from build123d import *

# Parameters (mm, degrees)
SKETCH1_R           = 9.8
SKETCH1_R_2         = 5
BOSS_EXTRUDE1_DEPTH = 10
SKETCH2_W           = 11.3
SKETCH2_H           = 11.3
CUT_EXTRUDE1_DEPTH  = 5
SKETCH3_W           = 11.313408722
SKETCH3_H           = 4.707055676
CUT_EXTRUDE2_DEPTH  = 3
SKETCH4_W           = 5.404805584
SKETCH4_H           = 18.076359344
SKETCH4_W_2         = 5.663408722
SKETCH4_H_2         = 17.947057775
CUT_EXTRUDE3_DEPTH  = 3
CHAMFER1_SIZE       = 3
CHAMFER2_SIZE       = 0.29
SKETCH5_R           = 12.8
SKETCH5_R_2         = 9.8
BOSS_EXTRUDE2_DEPTH = 1


with BuildPart() as part:
    # Sketch1 → Boss-Extrude1 (new body)
    with BuildSketch(Plane.XY):
        Circle(SKETCH1_R)
        Circle(SKETCH1_R_2, mode=Mode.SUBTRACT)
    extrude(amount=BOSS_EXTRUDE1_DEPTH)

    # Sketch2 → Cut-Extrude1 (cut)
    with BuildSketch(Plane.XY.offset(10)):
        Rectangle(SKETCH2_W, SKETCH2_H)
    extrude(amount=-CUT_EXTRUDE1_DEPTH, mode=Mode.SUBTRACT)

    # Sketch3 → Cut-Extrude2 (cut)
    with BuildSketch(Plane.XY.offset(10)):
        with Locations((0.006704361, 8.003527838)):
            Rectangle(SKETCH3_W, SKETCH3_H)
    extrude(amount=-CUT_EXTRUDE2_DEPTH, mode=Mode.SUBTRACT)

    # Sketch4 → Cut-Extrude3 (cut)
    with BuildSketch(Plane.XY.offset(10)):
        with Locations((-10.5897985, 0)):
            Rectangle(SKETCH4_W, SKETCH4_H)
        with Locations((10.615658814, 0.064650784)):
            Rectangle(SKETCH4_W_2, SKETCH4_H_2)
    extrude(amount=-CUT_EXTRUDE3_DEPTH, mode=Mode.SUBTRACT)

    # Chamfer1
    chamfer1_edges = [part.edges().sort_by_distance(p)[0] for p in [
        (-5, 0, 0),
    ]]
    chamfer(chamfer1_edges, length=CHAMFER1_SIZE)

    # Chamfer2
    chamfer2_edges = [part.edges().sort_by_distance(p)[0] for p in [
        (-9.8, 0, 0),
    ]]
    chamfer(chamfer2_edges, length=CHAMFER2_SIZE)

    # Sketch5 → Boss-Extrude2 (add)
    with BuildSketch(Plane(origin=(0, 0, 5), x_dir=(-1, 0, 0), z_dir=(0, 0, -1))):
        Circle(SKETCH5_R)
        Circle(SKETCH5_R_2, mode=Mode.SUBTRACT)
    extrude(amount=-BOSS_EXTRUDE2_DEPTH)


solid = part.part
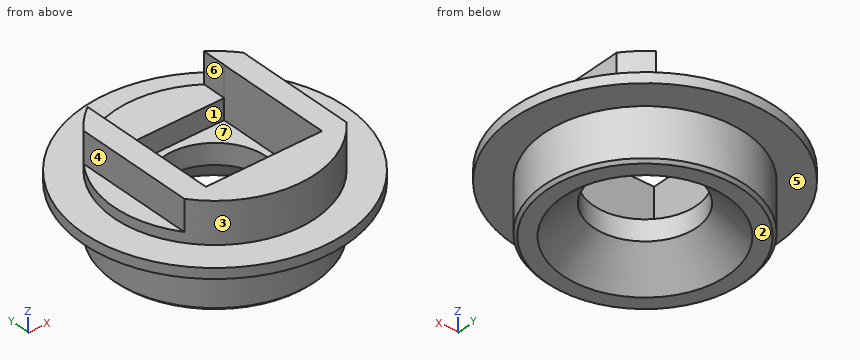
Build history of the part. All positions in model axes, mm. Face numbers are marked on the shaded views. A direction names the side the tool comes from. Give positions to 0.01 mm unless a question says otherwise; leave off trailing zeros. Loops run counter-clockwise (first coordinate to the right, second up) from the corner with the lowest first, then second, coordinate; pieces in that order, holes last. Notation, with made-up numbers: (4, -15.5) - (14, -15.5) arc R19 cw to (14, 10.5) - close; hole circle Ø8 at (68, 83). An arc over 180 degrees is marked (long way). Write item = value, one per line. Start each with the question number.
1) Band-saw the part on B-B on y = 0. Give the cut face in (x, z).
2) Tool access for the marked faces 5, 6 and 7: list every direction of +Z, -Z, +X, -X, +Y, -Y with a clear straight run to the whole face (end or side of a thin tool).
3) Pull direction X, two halves, no side cores. Call the marked faces 1, 2, 3 and 4: +X half, -X half, draft (parallel to the pull), parting line (faces both ways), or undercut.
4) Probe probe 1 along Y at (x, z) = (0, 3.95); probe 2 along X at (y, z) = (-4.75, 8.25); probe 3 along Z at (x, y) = (7.5, 8). List the from-to ranges inside material, lowest first. Write a range as from..to.
5) Drop flat-ended pins along their axis: pin 1 Ø1.5 at (y, z) = (1.5, 7.5) entering from +X; pin 2 Ø3.5 at (x, y) = (1.5, 8.5) entering from +Z; pin 3 Ø1.2 at (y, z) = (7, 8) entering from -X. Give the stop position or say it passes through.
6) Band-saw the part on A-A on x = 0. Give the cut face in (y, z), plus the area to 3 significant figures.
7) Band-saw the part on D-D on z = 1.5. Give the cut face in (x, y), plus the area to 3 significant figures.
Final values:
q1.outline = (-12.8, 5) - (-9.8, 5) - (-9.8, 0.29) - (-9.51, 0) - (-8, 0) - (-5, 3) - (-5, 5) - (-5.65, 5) - (-5.65, 10) - (-7.89, 10) - (-7.89, 7) - (-9.8, 7) - (-9.8, 6) - (-12.8, 6) - close; (5, 3) - (8, 0) - (9.51, 0) - (9.8, 0.29) - (9.8, 5) - (12.8, 5) - (12.8, 6) - (9.8, 6) - (9.8, 7) - (7.78, 7) - (7.78, 10) - (5.65, 10) - (5.65, 5) - (5, 5) - close
q2.face_5 = -Z
q2.face_6 = +Z, +Y
q2.face_7 = +Z
q3.face_1 = undercut
q3.face_2 = draft
q3.face_3 = parting line
q3.face_4 = -X half
q4.probe_1 = -9.8..-5, 5..9.8
q4.probe_2 = -7.89..-5.65, 5.65..7.78
q4.probe_3 = 5..6
q5.pin_1 = 9.75
q5.pin_2 = 7
q5.pin_3 = -7.42
q6.outline = (-12.8, 5) - (-9.8, 5) - (-9.8, 0.29) - (-9.51, 0) - (-8, 0) - (-5, 3) - (-5, 5) - (-5.65, 5) - (-5.65, 10) - (-9.8, 10) - (-9.8, 6) - (-12.8, 6) - close; (5, 3) - (8, 0) - (9.51, 0) - (9.8, 0.29) - (9.8, 5) - (12.8, 5) - (12.8, 6) - (9.8, 6) - (9.8, 7) - (5.65, 7) - (5.65, 5) - (5, 5) - close
q6.area = 74.0 mm²
q7.outline = circle Ø19.6 at (0, 0); hole circle Ø13 at (0, 0)
q7.area = 169 mm²
